Could you check a few things on this drawing? It's one solid part, dimensions in mm from its lowest x, y, z. A direction names the side the tool comes from. Round coordinates to 2 decimals unless told otherwise and drop trailing zeros. Write each loop counter-clockwise with the first axis right and the second up, starting at its lowest first coordinate (ties: lowest second). Pieces come first, ordered by that corner, then holes. Notation, with made-up numbers: (6.5, 3.5) -> (48.5, 3.5) arc R34 cw to (48.5, 42.5) -> close; hole circle Ø1 at (-24.5, -0.5). An arc over 180 degrees is marked (long way). Put each result on its own line as item: value. Start each with the question number.
1) I want a section at D-D, the plane x = 22.5. List the corners of the cut face in (y, z) for me (1 decimal), then the cut area to 3 significant figures.
2) If I drill on line 1 along X through (y, z) = (54.5, 6.25); line 2 along Z through (x, y) = (41, 70); line 3 along Y through (x, z) = (21, 13), over which ranges is the centre line in solid material (lowest first)? Write a range as [from, to].
3) Will these pins go through, and if not, where does the flat tip stop? P1, Ø2, axis at x = 40.5, z = 9.5, coming from the -Y side; P2, Ø6, axis at x = 8, z = 14.5, coming from the -Y side; P3, Ø6, axis at x = 24, y = 8.5, coming from the -Z side.
4) I want a section at B-B, the plane z = 10. Give the number of separate pieces and of enclosed holes in the cut face.
5) I want a section at A-A, the plane y = 62. List the corners of the cut face in (x, z) for me.
6) Which directions (+Z, -Z, +X, -X, +Y, -Y) give clear straight access to the entire face, cutting with the end or side of a thin tool? Please do the marked faces 1 and 2.
7) We'd pull the mould along Z, two halves only. Please class the marked faces 3, 4 and 5: released by +Z, released by -Z, zero draft, split by the parting line, or undercut.
8) I want a section at C-C, the plane y = 70. List the corners of the cut face in (x, z) for me.
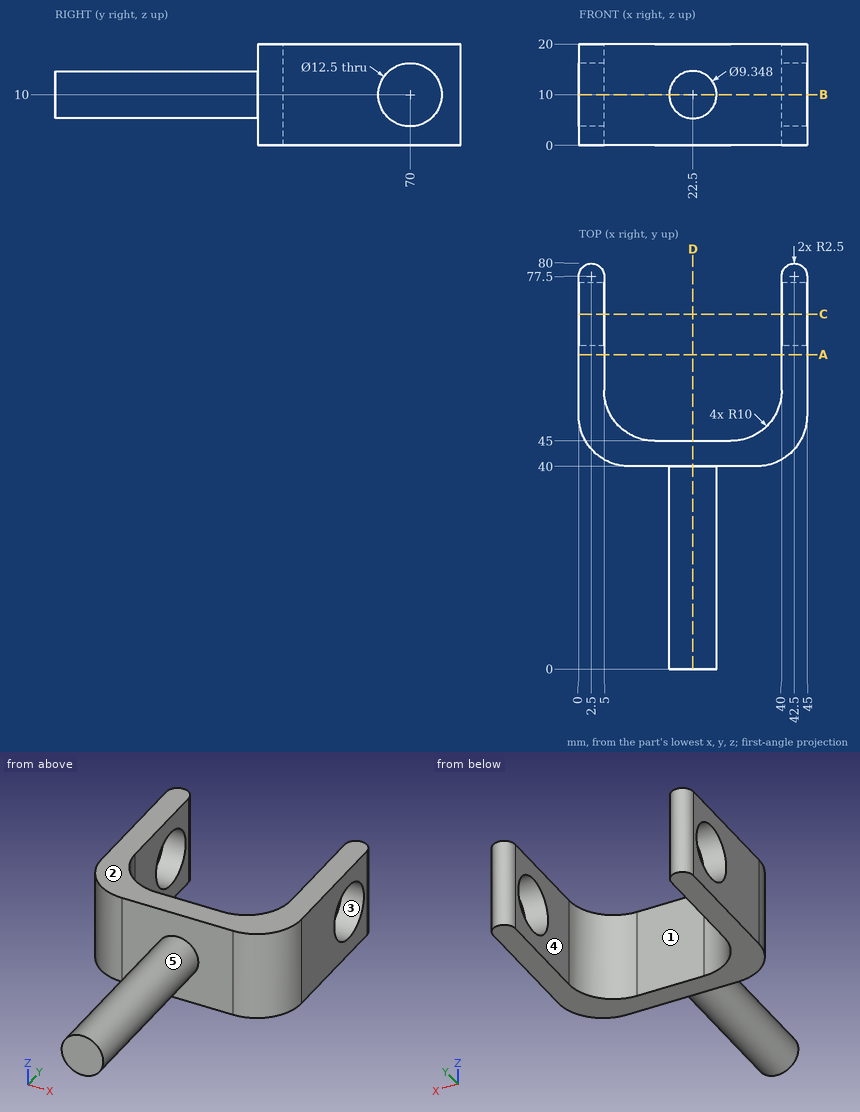
Findings:
1. outline: (0, 5.3) -> (40, 5.3) -> (40, 0) -> (45, 0) -> (45, 20) -> (40, 20) -> (40, 14.7) -> (0, 14.7) -> close
1. area: 474 mm2
2. line 1: x = [0, 5.01], [39.99, 45]
2. line 2: z = [0, 3.75], [16.25, 20]
2. line 3: y = [0, 45]
3. P1: stops at y = 41.07
3. P2: stops at y = 40
3. P3: stops at z = 5.33
4. separate pieces: 3
4. enclosed holes: 0
5. outline: (0, 0) -> (5, 0) -> (5, 20) -> (0, 20) -> close; (40, 0) -> (45, 0) -> (45, 20) -> (40, 20) -> close
6. face 1: +Z, -Z, +Y
6. face 2: +Z, +X, -X, +Y, -Y
7. face 3: undercut
7. face 4: zero draft
7. face 5: split by the parting line
8. outline: (0, 0) -> (5, 0) -> (5, 3.75) -> (0, 3.75) -> close; (0, 16.25) -> (5, 16.25) -> (5, 20) -> (0, 20) -> close; (40, 0) -> (45, 0) -> (45, 3.75) -> (40, 3.75) -> close; (40, 16.25) -> (45, 16.25) -> (45, 20) -> (40, 20) -> close
